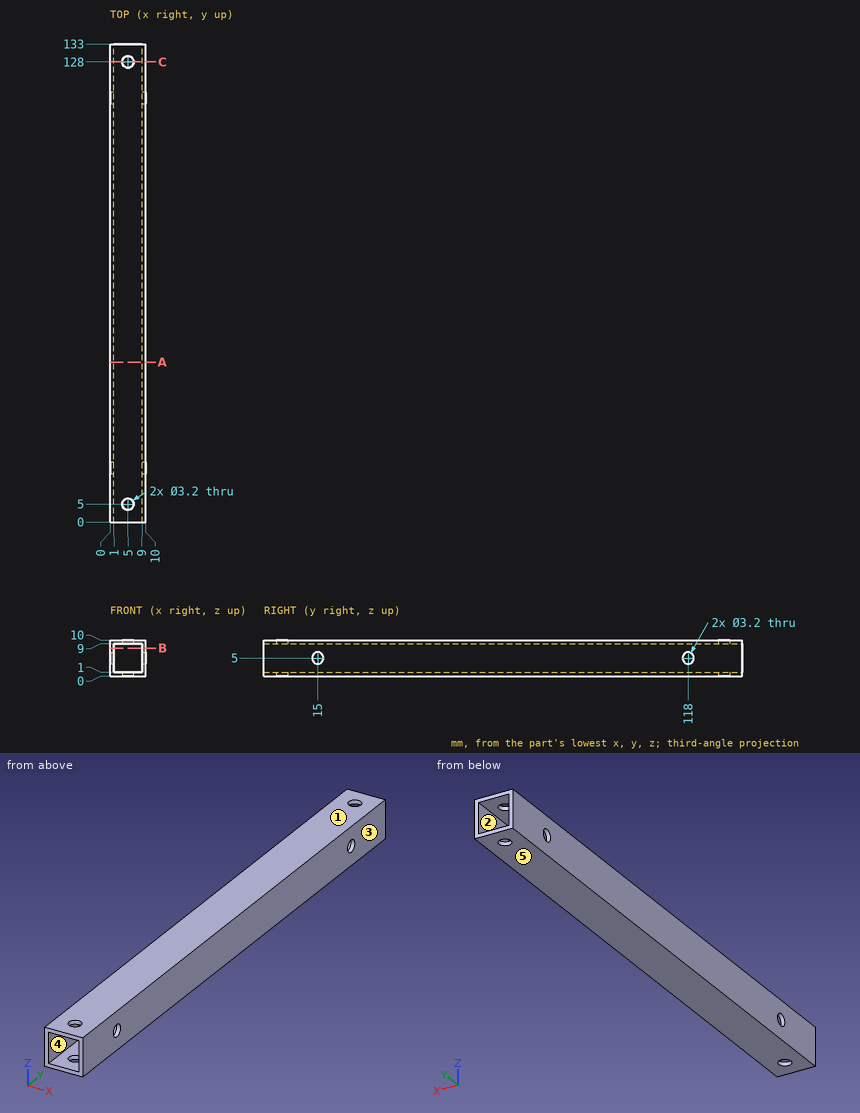
For this review, use the dimensioned drawing (mm, ordinates from the lowest corner) and the shaded views. A direction names the side the tool comes from. Coordinates: 2 decimals unless noted, no trailing zeros. Order: outer loops, then holes, each group sorted by start corner. A loop starts at its lowest first (then second) coordinate and runs counter-clockwise, first axis right, second up. Notation, with made-up numbers: (11.5, 16) -> (19.5, 16) arc R32 cw to (19.5, 54) -> close; hole circle Ø4 at (-32, -32.5). An arc over 180 degrees is marked (long way). One line per item, written item: value. Start each with the question number.
Q1. Take a section at C-C, the plane y = 128. State the section outline as (x, z) points, then the cut area to 3 significant figures.
Q2. Take a section at B-B, the plane z = 7.75. State the section outline as (x, y) points, then the cut area to 3 significant figures.
Q3. Tool access review of the marked faces 1 and 2: name each direction out of +Z, -Z, +X, -X, +Y, -Y from which nothing blocks a thin tool from reaching the whole face with its end or side.
Q4. Mouldability with a two-part tool opening along Z and no side actions: class the marked faces 3, 4 and 5 as pulls with the +Z half, pulls with the -Z half, needs draft (parallel to the pull), parting line crosses it, or undercut.
Q5. Insertion check: pin 1 Ø5 at (y, z) = (118, 5) entering from -X. The pin has a flat end and moves straight along its axis. Give the tip position at first contact, or say it passes through.
Q6. Take a section at A-A, the plane y = 44.5. State the section outline as (x, z) points.
Q7. For probe 1 along Y at (x, z) = (5, 0.8); probe 2 along X at (y, z) = (83, 4.5); probe 3 along Z at (x, y) = (0.3, 118), list the stretches that pass through material, from the lowest coordinate up.
Values follow:
1. outline: (0, 0) -> (3.4, 0) -> (3.4, 1) -> (1, 1) -> (1, 9) -> (3.4, 9) -> (3.4, 10) -> (0, 10) -> close; (6.6, 0) -> (10, 0) -> (10, 10) -> (6.6, 10) -> (6.6, 9) -> (9, 9) -> (9, 1) -> (6.6, 1) -> close
1. area: 29.6 mm2
2. outline: (0, 0) -> (1, 0) -> (1, 133) -> (0, 133) -> close; (9, 0) -> (10, 0) -> (10, 133) -> (9, 133) -> close
2. area: 266 mm2
3. face 1: +Z, +X, -X, +Y, -Y
3. face 2: +Y, -Y
4. face 3: needs draft
4. face 4: undercut
4. face 5: pulls with the -Z half
5. pin 1: stops at x = 0
6. outline: (0, 0) -> (10, 0) -> (10, 10) -> (0, 10) -> close; hole (1, 1) -> (9, 1) -> (9, 9) -> (1, 9) -> close
7. probe 1: y = 0 to 3.4, 6.6 to 126.4, 129.6 to 133
7. probe 2: x = 0 to 1, 9 to 10
7. probe 3: z = 0 to 3.4, 6.6 to 10
